from build123d import *

# Parameters (mm, degrees)
F1_DEPTH = 2
F3_DEPTH = 50


with BuildPart() as f1:
    # F0 (on Top) → F1 (new body)
    with BuildSketch(Plane.XY):
        Polygon((60, 60), (-60, 60), (-60, -60), (-40, -60), (60, 40), align=None)
    extrude(amount=F1_DEPTH)

    # F2 (on face) → F3 (join)
    with BuildSketch(Plane.XY.offset(2)):
        Polygon((60, 55), (60, 60), (-60, 60), (-60, 55), (-60, -60), (-55, -60), (-55, 55), align=None)
    extrude(amount=F3_DEPTH)


solid = f1.part
Design review of the part built by this model. Coordinates are the model's own, in mm. A direction names the side the tool comes from. Coordinates: 2 decimals unless noted, no trailing zeros. Write each loop counter-clockwise with the first axis right and the second up, starting at its lowest first coordinate (ties: lowest second). Pieces come first, ordered by that corner, then holes. Notation, with made-up numbers: (30, -34.75) - (47, -34.75) arc R24 cw to (47, -8.75) - close; hole circle Ø11 at (13, 38.5). An arc over 180 degrees is marked (long way). One line per item, written item: value.
1) To check wall thickness, follow probe 1 along X at (y, z) = (0, 12.5); probe 2 along Y at (x, z) = (5, 34); probe 3 along Z at (x, y) = (-27.5, -13). State the ranges of each line that lie inside material, in increasing order.
Answer sheet:
probe 1: x = -60 to -55
probe 2: y = 55 to 60
probe 3: z = 0 to 2
2) Add section B-B (y = -16). State the section outline as (x, z) points.
Answer sheet:
outline: (-60, 0) - (4, 0) - (4, 2) - (-55, 2) - (-55, 52) - (-60, 52) - close
3) For faces 1 (the face through (-14, 14, 0)), 2 (the face through (2, 55, 27)), list the 3-axis set-ups (+Z, -Z, +X, -X, +Y, -Y) from which the entire face can be reached by the end or side of a thin tool; tool diameter is ignored.
Answer sheet:
face 1: -Z, +X, -X, +Y, -Y
face 2: +Z, +X, -Y
4) Insertion check: pin 1 (3 mm diameter, centred on x = -15, y = 4, fed in from +Z); pin 2 (1.5 mm diameter, centred on y = -26, z = 35.5, fed in from +X); pin 3 (2 mm diameter, centred on x = -4.5, z = 47, fed in from -Y). Each pin has a flat end and moves straight along its axis. Give the tip position at first contact, or say it passes through.
Answer sheet:
pin 1: stops at z = 2
pin 2: stops at x = -55
pin 3: stops at y = 55
5) Add section A-A (x = -46). State the section outline as (y, z) points, plus the area to 3 significant figures.
Answer sheet:
outline: (-60, 0) - (60, 0) - (60, 52) - (55, 52) - (55, 2) - (-60, 2) - close
area: 490 mm2
